from build123d import *

# Parameters (mm, degrees)
F1_DEPTH      = 7.9375
F1_DEPTH_BACK = 7.9375
F4_R          = 2.55
F5_DEPTH      = 25.4
F5_DEPTH_BACK = 25.4
F6_START      = 1.5875
F4_R_2        = 4.25
F6_DEPTH      = 23.8125


with BuildPart() as f1:
    # F0 (on Front) → F1 (new body, two sides)
    with BuildSketch(Plane.XZ) as f1_sk:
        Polygon((-13.97, 0), (0, 0), (2.1268467149, 7.9375), (-14.6644412667, 7.9375), align=None)
    extrude(amount=F1_DEPTH)
    extrude(f1_sk.sketch, amount=-F1_DEPTH_BACK)

    # F4 (on line) → F5 (cut, two sides)
    with BuildSketch(Plane(origin=(0, 0, 0), x_dir=(0.9518743809, 0, -0.3064884386), z_dir=(0.3064884386, 0, 0.9518743809))) as f5_sk:
        with Locations((-8.4281116724, 0)):
            Circle(F4_R)
    extrude(amount=-F5_DEPTH, mode=Mode.SUBTRACT)
    extrude(f5_sk.sketch, amount=F5_DEPTH_BACK, mode=Mode.SUBTRACT)

    # F4 (on line) → F6 (cut)
    with BuildSketch(Plane(origin=(0, 0, 0), x_dir=(0.9518743809, 0, -0.3064884386), z_dir=(0.3064884386, 0, 0.9518743809)).offset(F6_START)):
        with Locations((-8.4281116724, 0)):
            Circle(F4_R_2)
        with Locations((-8.4281116724, 0)):
            Circle(F4_R, mode=Mode.SUBTRACT)
    extrude(amount=F6_DEPTH, mode=Mode.SUBTRACT)


solid = f1.part
Work out the finished part from the listing and answer in its coordinate system (mm). A direction names the side the tool comes from. Give positions to 0.01 mm unless a question says otherwise; leave off trailing zeros. Order: outer loops, then holes, each group sorted by start corner. A loop starts at its lowest first (then second) coordinate and runs counter-clockwise, first axis right, second up. Notation, with made-up numbers: (62.25, 12) -> (68.25, 12) arc R26 ccw to (68.25, 50) -> close; hole circle Ø7 at (-25, 45). An arc over 180 degrees is marked (long way). Answer as a JSON object with one key per item and string values. Group by question number.
1. Section B-B on y = 5 is taken. Determine the outline of the cut face in (x, z), plus the area to 3 significant figures.
2. Section A-A on y = -0.25 is taken. Determine the outline of the cut face in (x, z).
3. The mould has two halves that part along Y. Classify faces 3 (the cylindrical face through (-10.57, 0.11, 2.98)), 4 (the flat face through (-6, -7.938, 4)), 5 (the flat face through (1.049, -0.111, 3.913)), 6 (the cylindrical face through (-3.045, 1.277, 4.817)): released by +Y, released by -Y, zero draft, split by the parting line, or undercut.
4. Section C-C on y = -2 is taken. Determine the outline of the cut face in (x, z), plus the area to 3 significant figures.
5. A tool of negligible diameter and unlimited length cuts with its end or side. For faces 1 (the flat face through (-6, 0, 0)), 2 (the flat face through (-4.896, 0.06, 3.244)), from which of +Z, -Z, +X, -X, +Y, -Y can it reach the whole face along a straight path? Write none if from no direction.
6. Consider line 1 along Y through (x, z) = (-4.25, 7.5); line 2 along X through (y, z) = (0, 3.75); line 3 along Y through (x, z) = (-10, 3.75). Determine where each line is inside the solid, lowest interval first. Write a range as [from, to].
7. Flat-ended cylindrical pins translate along their axes: pin 1 Ø5 at (x, y) = (-10, 0.5) entering from -Z; pin 2 Ø1.5 at (y, z) = (3.5, 7) entering from +X; pin 3 Ø3 at (y, z) = (2, 4) entering from +X. Find the tip coordinate at first contact, or state that the pin passes through.
Result sheet:
{
 "1": {"outline": "(-14.66, 7.94) -> (-13.97, 0) -> (0, 0) -> (2.13, 7.94) -> close", "area": "122 mm^2"},
 "2": {"outline": "(-14.66, 7.94) -> (-13.97, 0) -> (-11.52, 0) -> (-9.95, 4.87) -> (-11.57, 5.39) -> (-10.76, 7.94) -> close; (-6.19, 0) -> (0, 0) -> (2.13, 7.94) -> (-1.84, 7.94) -> (-3.5, 2.79) -> (-5.12, 3.32) -> close"},
 "3": {"face 3": "undercut", "face 4": "released by -Y", "face 5": "zero draft", "face 6": "undercut"},
 "4": {"outline": "(-14.66, 7.94) -> (-13.97, 0) -> (-10.52, 0) -> (-9.04, 4.58) -> (-11.11, 5.24) -> (-10.24, 7.94) -> close; (-7.19, 0) -> (0, 0) -> (2.13, 7.94) -> (-2.36, 7.94) -> (-3.97, 2.94) -> (-6.03, 3.61) -> close", "area": "78.2 mm^2"},
 "5": {"face 1": "-Z, +X, -X, +Y, -Y", "face 2": "none"},
 "6": {"line 1": "y = [-7.94, -3.7], [3.7, 7.94]", "line 2": "x = [-14.3, -10.33], [-3.18, 1]", "line 3": "y = [-7.94, -1.22], [1.22, 7.94]"},
 "7": {"pin 1": "stops at z = 0", "pin 2": "stops at x = 2.08", "pin 3": "stops at x = 1.47"}
}
